from build123d import *

# Parameters (mm, degrees)
F0_R           = 30
F1_DEPTH       = 20
F2_R           = 21.9
F3_DEPTH       = 5
F4_R           = 20
F5_DEPTH       = 42
F6_R           = 21.9
F7_DEPTH       = 3
F10_DEPTH      = 75
F11_R          = 4
F12_DEPTH      = 100
F12_DEPTH_BACK = 100
F13_R          = 4
F14_DEPTH      = 100
F14_DEPTH_BACK = 100


# Not quite as in the source:
# - a fillet or chamfer that OpenCascade refuses, or shapes differently, is made with other operations: its cross-section is extruded or revolved along the edge and cut away or added


with BuildPart() as f1:
    # F0 (on Top) → F1 (new body)
    with BuildSketch(Plane.XY):
        Circle(F0_R)
    extrude(amount=F1_DEPTH)

    # F2 (on face) → F3 (join)
    with BuildSketch(Plane.XY.offset(20)):
        Circle(F2_R)
    extrude(amount=F3_DEPTH)

    # F4 (on face) → F5 (join)
    with BuildSketch(Plane.XY.offset(25)):
        Circle(F4_R)
    extrude(amount=F5_DEPTH)

    # F6 (on face) → F7 (join)
    with BuildSketch(Plane.XY.offset(67)):
        Circle(F6_R)
    extrude(amount=F7_DEPTH)

    # F8: fillet of radius 2 on 1 edges, made by hand

    # F8_s1 → F8_t2 (revolve, cut)
    with BuildSketch(Plane.XZ):
        with BuildLine():
            ThreePointArc((20, 25), (21.3491376746, 24.3809064397), (21.9, 23.0025015645))
            Line((21.9, 23.0025015645), (21.9, 25))
            Line((21.9, 25), (20, 25))
        make_face()
    revolve(axis=Axis((0, 0, 25), (0, 0, 1)), mode=Mode.SUBTRACT)

    # F9 (on face) → F10 (cut)
    with BuildSketch(Plane.XY.offset(70)):
        with BuildLine():
            Line((18, 4), (14.4568322948, 4))
            ThreePointArc((14.4568322948, 4), (-2.0183552187, 14.8635877974), (-15, 0))
            Line((-15, 0), (0, 0))
            Line((0, 0), (15, 0))
            Line((15, 0), (18, 0))
            Line((18, 0), (18, 4))
        make_face()
        with BuildLine():
            Line((0, 0), (-15, 0))
            ThreePointArc((-15, 0), (-2.0183552187, -14.8635877974), (14.4568322948, -4))
            Line((14.4568322948, -4), (18, -4))
            Line((18, -4), (18, 0))
            Line((18, 0), (15, 0))
            Line((15, 0), (0, 0))
        make_face()
    extrude(amount=-F10_DEPTH, mode=Mode.SUBTRACT)

    # F11 (on Right) → F12 (cut, two sides)
    with BuildSketch(Plane.YZ) as f12_sk:
        with Locations((0, 10)):
            Circle(F11_R)
    extrude(amount=F12_DEPTH, mode=Mode.SUBTRACT)
    extrude(f12_sk.sketch, amount=-F12_DEPTH_BACK, mode=Mode.SUBTRACT)

    # F13 (on Front) → F14 (cut, two sides)
    with BuildSketch(Plane.XZ) as f14_sk:
        with Locations((0, 10)):
            Circle(F13_R)
    extrude(amount=-F14_DEPTH, mode=Mode.SUBTRACT)
    extrude(f14_sk.sketch, amount=F14_DEPTH_BACK, mode=Mode.SUBTRACT)


solid = f1.part
Check sheet for the modelled part. Datum: model origin and axes. Units: mm. A direction names the side the tool comes from. Give positions to 0.01 mm unless a question says otherwise; leave off trailing zeros. Order: outer loops, then holes, each group sorted by start corner. A loop starts at its lowest first (then second) coordinate and runs counter-clockwise, first axis right, second up. Notation, with made-up numbers: M 68,22 L 123,22 A29 ccw 123,50 Z; hole C 24.5,84 d1. An arc over 180 degrees is marked long. Answer as CSV lines item,"result". Start each with the question number.
Item 1: Gauge pin test, flat ends, axial feed: P1, Ø3, axis at x = 16.5, z = 40.5, coming from the +Y side; P2, Ø4, axis at x = 7.5, z = 18.5, coming from the +Y side; P3, Ø2.5, axis at y = -1, z = 4.5, coming from the -X side; P4, Ø1.5, axis at x = -1.5, z = 15.5, coming from the +Y side. Record the tip position at first contact, or that the pin passes through.
Item 2: Mould release check, pull along Y, two halves, no side actions. Record for faces 4 (the face through (-0.521, -22.124, 13.966)), 5 (the face through (18, 0, 3)), 6 (the face through (16, -4, 35)), 7 (the face through (-17.4, -13.3, 68.5)): +Y half, -Y half, draft (parallel to the pull), parting line (faces both ways), or undercut.
Item 3: Cross-section at D-D on z = 8. Enter the section's corners in (x, y), plus the area to 3 significant figures.
Item 4: Cross-section at B-B on x = 0. Enter the section's corners in (y, z).
Item 5: Thickness scan on line 1 (X direction, y = 0.5, z = 65); line 2 (Z direction, x = 23.25, y = 0); line 3 (Y direction, x = 0, z = 39). Record the ranges inside material, lowest first. Write a range as [from, to].
Item 6: Tool access check on faces 1 (the face through (2, -22, 20)), 2 (the face through (16, 4, 35)), 3 (the face through (-4.336, -19.524, 45.706)). Record the directions out of +Z, -Z, +X, -X, +Y, -Y that give a thin tool (end or side, any length) a straight path to the whole face; none if there is none.
Item 7: Cross-section at C-C on z = 37.5. Enter the section's corners in (x, y).
Item 8: Cross-section at A-A on y = 0. Enter the section's corners in (x, z), plus the area to 3 significant figures.
Established:
1,P1,"stops at y = 13.23"
1,P2,"stops at y = 29.49"
1,P3,"stops at x = -30"
1,P4,"stops at y = 29.99"
2,face 4,"draft"
2,face 5,"undercut"
2,face 6,"undercut"
2,face 7,"parting line"
3,outline,"M -29.8,-3.46 A30 ccw -3.46,-29.8 L -3.46,-14.59 A15 cw -14.59,-3.46 Z; M -29.8,3.46 L -14.59,3.46 A15 cw -3.46,14.59 L -3.46,29.8 A30 ccw Z; M 3.46,-29.8 A30 ccw 29.8,-3.46 L 18,-3.46 L 18,-4 L 14.46,-4 A15 cw 3.46,-14.59 Z; M 3.46,14.59 A15 cw 14.46,4 L 18,4 L 18,3.46 L 29.8,3.46 A30 ccw 3.46,29.8 Z"
3,area,"1,700 mm^2"
4,outline,"M -30,0 L -15,0 L -15,6 L -30,6 Z; M -30,14 L -15,14 L -15,70 L -21.9,70 L -21.9,67 L -20,67 L -20,25 A2 ccw -21.9,23 L -21.9,20 L -30,20 Z; M 15,0 L 30,0 L 30,6 L 15,6 Z; M 15,14 L 30,14 L 30,20 L 21.9,20 L 21.9,23 A2 ccw 20,25 L 20,67 L 21.9,67 L 21.9,70 L 15,70 Z"
5,line 1,"x = [-19.99, -14.99], [18, 19.99]"
5,line 2,"z = [0, 6], [14, 20]"
5,line 3,"y = [-20, -15], [15, 20]"
6,face 1,"+Z"
6,face 2,"+Z, -Z"
6,face 3,"none"
7,outline,"C 0,0 d40; hole M 14.46,-4 L 18,-4 L 18,4 L 14.46,4 A15 ccw long Z"
8,outline,"M -30,0 L -15,0 L -15,6 L -30,6 Z; M -30,14 L -15,14 L -15,70 L -21.9,70 L -21.9,67 L -20,67 L -20,25 A2 ccw -21.9,23 L -21.9,20 L -30,20 Z; M 18,0 L 30,0 L 30,6 L 18,6 Z; M 18,14 L 30,14 L 30,20 L 21.9,20 L 21.9,23 A2 ccw 20,25 L 20,67 L 21.9,67 L 21.9,70 L 18,70 Z"
8,area,"703 mm^2"
